Print and shaded views of the part. All mm, measured from the part's lowest x, y and z. Give positions to 0.01 mm unless a question says otherwise; leave off trailing zeros. Order: outer loops, then holes, each group sorted by start corner. A loop starts at its lowest first (then second) coordinate and runs counter-clockwise, first axis right, second up. Notation, with made-up numbers: (60.25, 19.5) - (99.25, 19.5) arc R29 cw to (99.25, 50.5) - close; hole circle Ø3 at (-31.75, 66.25). An arc over 180 degrees is marked (long way). Answer in a Markdown table with one row per item.
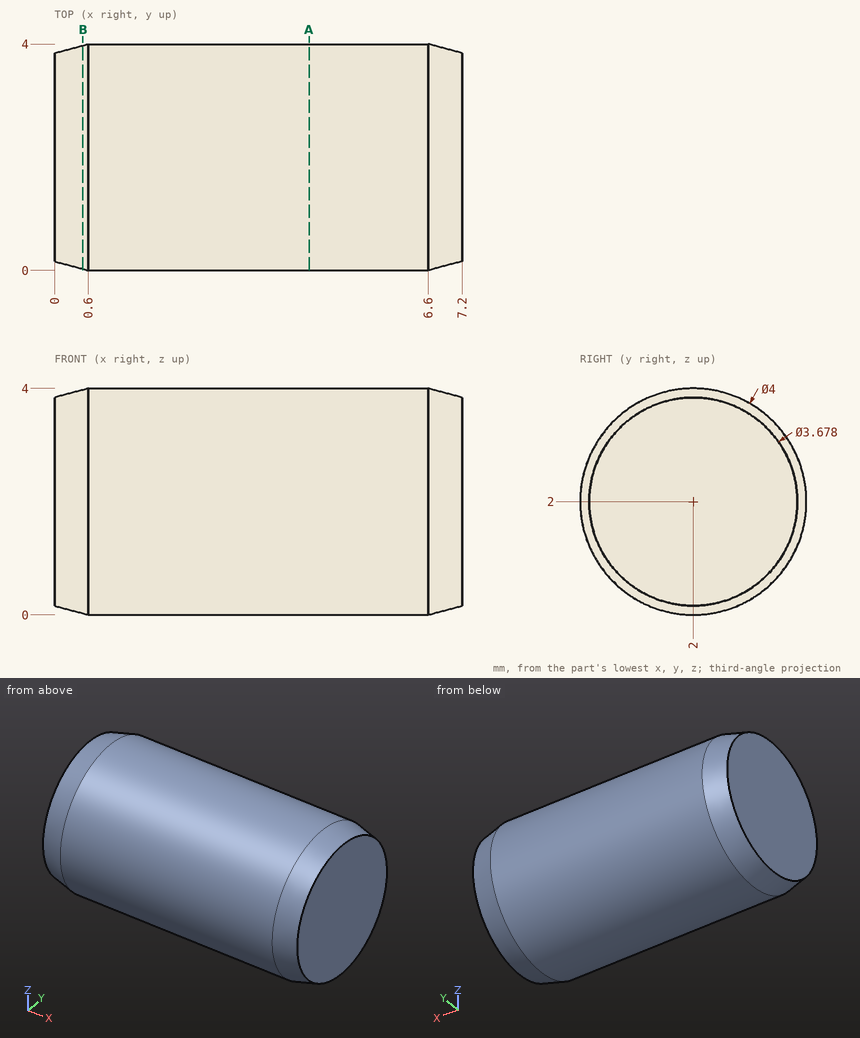
1. Probe line 1 (Z direction, x = 1.5, y = 2.65); line 2 (Y direction, x = 0.5, z = 1.95); line 3 (Y direction, x = 6, z = 2.6). List the from-to ranges inside material, lowest first.
Check result:
| item | result |
|---|---|
| line 1 | z = 0.11 to 3.89 |
| line 2 | y = 0.03 to 3.97 |
| line 3 | y = 0.09 to 3.91 |
2. Cut at A-A on x = 4.5. Write the cut outline in (y, z).
Check result:
| item | result |
|---|---|
| outline | circle Ø4 at (2, 2) |
3. Cut at B-B on x = 0.5. Write the cut outline in (y, z).
Check result:
| item | result |
|---|---|
| outline | circle Ø3.95 at (2, 2) |
4. Drop a flat-ended pin along its axis: P1, Ø1.5, axis at x = 2.5, y = 3, coming from the +Z side. Give the stop position or say it passes through.
Check result:
| item | result |
|---|---|
| P1 | stops at z = 3.98 |
